```python
from build123d import *

# Parameters (mm, degrees)
EXTRUDE_1_DEPTH      = 15
EXTRUDE_1_DEPTH_BACK = 15
SKETCH_3_W           = 52
SKETCH_3_H           = 52
CUT_EXTRUDE_1_DEPTH  = 26.5
FILLET_1_R           = 2
SKETCH_4_R           = 4.5
CUT_EXTRUDE_2_DEPTH  = 7
SKETCH_5_R           = 4.5
CUT_EXTRUDE_3_DEPTH  = 7
SKETCH_6_W           = 5
SKETCH_6_H           = 49.5
SKETCH_6_W_2         = 9
SKETCH_6_H_2         = 42
CUT_EXTRUDE_4_DEPTH  = 3
SKETCH_7_W           = 49.5
SKETCH_7_H           = 5
SKETCH_7_W_2         = 42
SKETCH_7_H_2         = 9
CUT_EXTRUDE_5_DEPTH  = 3
SKETCH_8_W           = 3
SKETCH_8_H           = 8
EXTRUDE_2_DEPTH      = 2
SKETCH_9_W           = 8
SKETCH_9_H           = 3
EXTRUDE_3_DEPTH      = 2


with BuildPart() as part:
    # Sketch 2 → Extrude 1 (new body, two sides)
    with BuildSketch(Plane.XY) as extrude_1_sk:
        Polygon((0, 58), (0, 0), (58, 0), (58, 12), (52, 12), (12, 52), (12, 58), align=None)
    extrude(amount=EXTRUDE_1_DEPTH)
    extrude(extrude_1_sk.sketch, amount=-EXTRUDE_1_DEPTH_BACK)

    # Sketch 3 → Cut-Extrude 1 (cut)
    with BuildSketch(Plane.XY.offset(15)):
        with Locations((32, 32)):
            Rectangle(SKETCH_3_W, SKETCH_3_H)
    extrude(amount=-CUT_EXTRUDE_1_DEPTH, mode=Mode.SUBTRACT)

    # Fillet 1
    fillet_1_edges = [part.edges().sort_by_distance(p)[0] for p in [
        (12, 58, -13.25),
        (12, 52, -13.25),
        (52, 12, -13.25),
        (58, 12, -13.25),
    ]]
    fillet(fillet_1_edges, radius=FILLET_1_R)

    # Sketch 4 → Cut-Extrude 2 (cut, through all)
    with BuildSketch(Plane(origin=(6, 0, 0), x_dir=(0, 0, -1), z_dir=(1, 0, 0))):
        with Locations(Location((0, 42.5, 0), (0, 0, 90))):  # turned: the seam where the file's is
            Circle(SKETCH_4_R)
        with BuildLine():
            Line((4.5, 26.3), (4.5, 15.3))
            ThreePointArc((4.5, 15.3), (0, 10.8), (-4.5, 15.3))
            Line((-4.5, 15.3), (-4.5, 26.3))
            ThreePointArc((-4.5, 26.3), (0, 30.8), (4.5, 26.3))
        make_face()
    extrude(amount=-CUT_EXTRUDE_2_DEPTH, mode=Mode.SUBTRACT)

    # Sketch 5 → Cut-Extrude 3 (cut, through all)
    with BuildSketch(Plane(origin=(0, 6, 0), x_dir=(1, 0, 0), z_dir=(0, 1, 0))):
        with Locations(Location((42.5, 0, 0), (0, 0, 270))):  # turned: the seam where the file's is
            Circle(SKETCH_5_R)
        with BuildLine():
            Line((15.3, 4.5), (26.3, 4.5))
            ThreePointArc((26.3, 4.5), (30.8, 0), (26.3, -4.5))
            Line((26.3, -4.5), (15.3, -4.5))
            ThreePointArc((15.3, -4.5), (10.8, 0), (15.3, 4.5))
        make_face()
    extrude(amount=-CUT_EXTRUDE_3_DEPTH, mode=Mode.SUBTRACT)

    # Sketch 6 → Cut-Extrude 4 (cut)
    with BuildSketch(Plane.ZY):
        with Locations((-9.25, 29.75)):
            Rectangle(SKETCH_6_W, SKETCH_6_H)
        with Locations((9.25, 29.75)):
            Rectangle(SKETCH_6_W, SKETCH_6_H)
        with Locations((0, 30)):
            Rectangle(SKETCH_6_W_2, SKETCH_6_H_2)
    extrude(amount=-CUT_EXTRUDE_4_DEPTH, mode=Mode.SUBTRACT)

    # Sketch 7 → Cut-Extrude 5 (cut)
    with BuildSketch(Plane.XZ):
        with Locations((29.75, 9.3)):
            Rectangle(SKETCH_7_W, SKETCH_7_H)
        with Locations((29.75, -9.3)):
            Rectangle(SKETCH_7_W, SKETCH_7_H)
        with Locations((30, 0)):
            Rectangle(SKETCH_7_W_2, SKETCH_7_H_2)
    extrude(amount=-CUT_EXTRUDE_5_DEPTH, mode=Mode.SUBTRACT)

    # Sketch 8 → Extrude 2 (add)
    with BuildSketch(Plane.XZ):
        with Locations((7.5, 0)):
            Rectangle(SKETCH_8_W, SKETCH_8_H)
        with Locations((52.5, 0)):
            Rectangle(SKETCH_8_W, SKETCH_8_H)
    extrude(amount=EXTRUDE_2_DEPTH)

    # Sketch 9 → Extrude 3 (add)
    with BuildSketch(Plane.ZY):
        with Locations((0, 52.5)):
            Rectangle(SKETCH_9_W, SKETCH_9_H)
        with Locations((0, 7.5)):
            Rectangle(SKETCH_9_W, SKETCH_9_H)
    extrude(amount=EXTRUDE_3_DEPTH)


solid = part.part
```
Geometry check sheet. Reference: the model listing, model coordinates, mm. A direction names the side the tool comes from. Coordinates: 2 decimals unless noted, no trailing zeros. Order: outer loops, then holes, each group sorted by start corner. A loop starts at its lowest first (then second) coordinate and runs counter-clockwise, first axis right, second up.
Q1. Sectioned sample at B-B on x = 27.5. Record the cut outline in (y, z).
Reply:
outline: (0, -15) - (36.5, -15) - (36.5, -11.5) - (6, -11.5) - (6, -4.34) - (3, -4.34) - (3, -4.5) - (0, -4.5) - (0, -6.8) - (3, -6.8) - (3, -11.8) - (0, -11.8) - close; (0, 4.5) - (3, 4.5) - (3, 4.34) - (6, 4.34) - (6, 15) - (0, 15) - (0, 11.8) - (3, 11.8) - (3, 6.8) - (0, 6.8) - close
Q2. Sectioned sample at C-C on y = 36. Record the cut outline in (x, z).
Reply:
outline: (0, -15) - (28, -15) - (28, -11.5) - (6, -11.5) - (6, 15) - (0, 15) - (0, 11.75) - (3, 11.75) - (3, 6.75) - (0, 6.75) - (0, 4.5) - (3, 4.5) - (3, -4.5) - (0, -4.5) - (0, -6.75) - (3, -6.75) - (3, -11.75) - (0, -11.75) - close
Q3. Draft check along X on faces 6 (the face through (0, 9, 0)), 7 (the face through (3, 30, -9)), 8 (the face through (29, 3, 9)). Enter one of: released by +X, released by -X, zero draft, split by the parting line, or undercut.
Reply:
face 6: zero draft
face 7: released by -X
face 8: undercut
Q4. Sectioned sample at D-D on z = 0. Give the number of separate pieces and of enclosed holes in the cut face, and give its area (3 significant figures).
Reply:
separate pieces: 5
enclosed holes: 0
area: 258 mm2
Q5. Thickness scan on probe 1 along Y at (x, z) = (5.05, 0); probe 2 along Z at (x, y) = (42.5, 5.2). Record the ranges inside material, lowest first.
Reply:
probe 1: y = 0 to 10.8, 30.8 to 38, 47 to 58
probe 2: z = -15 to -4.5, 4.5 to 15
Q6. Depth check by flat-ended pin: pin 1 Ø6 at (y, z) = (37, -11.5) entering from -X; pin 2 Ø0.6 at (x, y) = (-0.5, 7) entering from +Z; pin 3 Ø1.5 at (x, z) = (0.5, -1) entering from -Y. Enter the tip coordinate at first touch or a pass-through.
Reply:
pin 1: stops at x = 0
pin 2: stops at z = 4
pin 3: stops at y = 0
Q7. Tool access check on faces 1 (the face through (3, 35, 0)), 2 (the face through (-1, 7, -4)), 3 (the face through (32, 6, 2)), 4 (the face through (30.8, 4.5, -0.1)), 5 (the face through (-1, 7, 4)). Record the directions out of +Z, -Z, +X, -X, +Y, -Y that give a thin tool (end or side, any length) a straight path to the whole face; none if there is none.
Reply:
face 1: -X
face 2: -Z, -X, +Y, -Y
face 3: +Z, +X, +Y
face 4: +Y, -Y
face 5: +Z, -X, +Y, -Y
